For this review, use the dimensioned drawing (mm, ordinates from the lowest corner) and the shaded views. Coordinates: 2 decimals unless noted, no trailing zeros. Loops run counter-clockwise (first coordinate to the right, second up) from the corner with the lowest first, then second, coordinate; pieces in that order, holes last. Notation, with made-up numbers: M 56.5,-31.5 L 71.5,-31.5 A29 cw 71.5,-9.5 Z; hole C 76,-19.5 d11. An arc over 180 degrees is marked long. Use CSV: the item, a comma, the result in double quotes. Start each with the question number.
1. For L1, parallel to X at y = 180, z = 3.05; L2, parallel to Y at x = 109, z = 1.2; L3, parallel to X at y = 177, z = 3.65, list the stretches that pass through material, from the lowest coordinate up.
2. Clearance check with flat-ended pins moving along their axes: P1, Ø14.5, axis at x = 109, y = 180, coming from the +Z side; P2, Ø1.8, axis at x = 97.5, z = 4.5, coming from the +Y side. State where each tip first meets the part, or that it passes through.
3. Add section A-A, the plane y = 180. Write out the cut boundary in (x, z).
4. Add section C-C, the plane x = 105.5. Write out the cut boundary in (y, z).
5. Add section D-D, the plane x = 10. Write out the cut boundary in (y, z), then the cut area to 3 significant figures.
6. Add section B-B, the plane z = 4.45. Write out the cut boundary in (x, y), then the cut area to 3 significant figures.
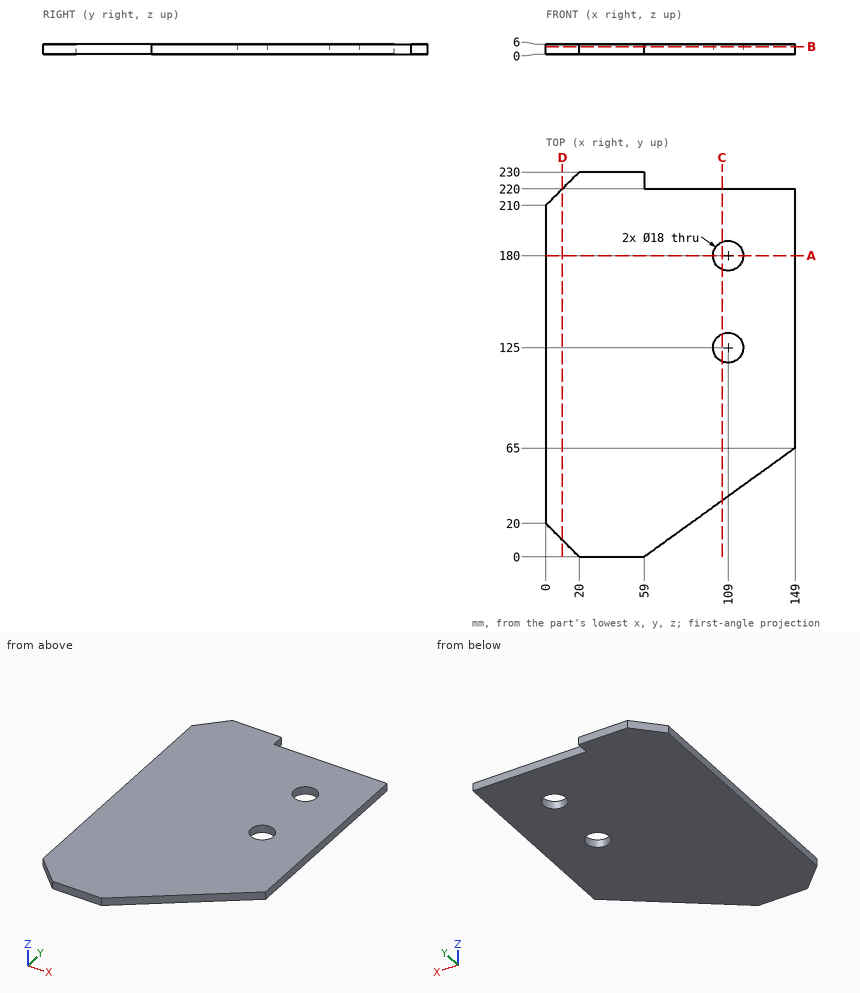
Computed:
1,L1,"x = 0 to 100, 118 to 149"
1,L2,"y = 36.11 to 116, 134 to 171, 189 to 220"
1,L3,"x = 0 to 100.51, 117.49 to 149"
2,P1,"passes through"
2,P2,"stops at y = 220"
3,outline,"M 0,0 L 100,0 L 100,6 L 0,6 Z; M 118,0 L 149,0 L 149,6 L 118,6 Z"
4,outline,"M 33.58,0 L 116.71,0 L 116.71,6 L 33.58,6 Z; M 133.29,0 L 171.71,0 L 171.71,6 L 133.29,6 Z; M 188.29,0 L 220,0 L 220,6 L 188.29,6 Z"
5,outline,"M 10,0 L 220,0 L 220,6 L 10,6 Z"
5,area,"1,260 mm^2"
6,outline,"M 0,20 L 20,0 L 59,0 L 149,65 L 149,220 L 59,220 L 59,230 L 20,230 L 0,210 Z; hole C 109,125 d18; hole C 109,180 d18"
6,area,"29,500 mm^2"
